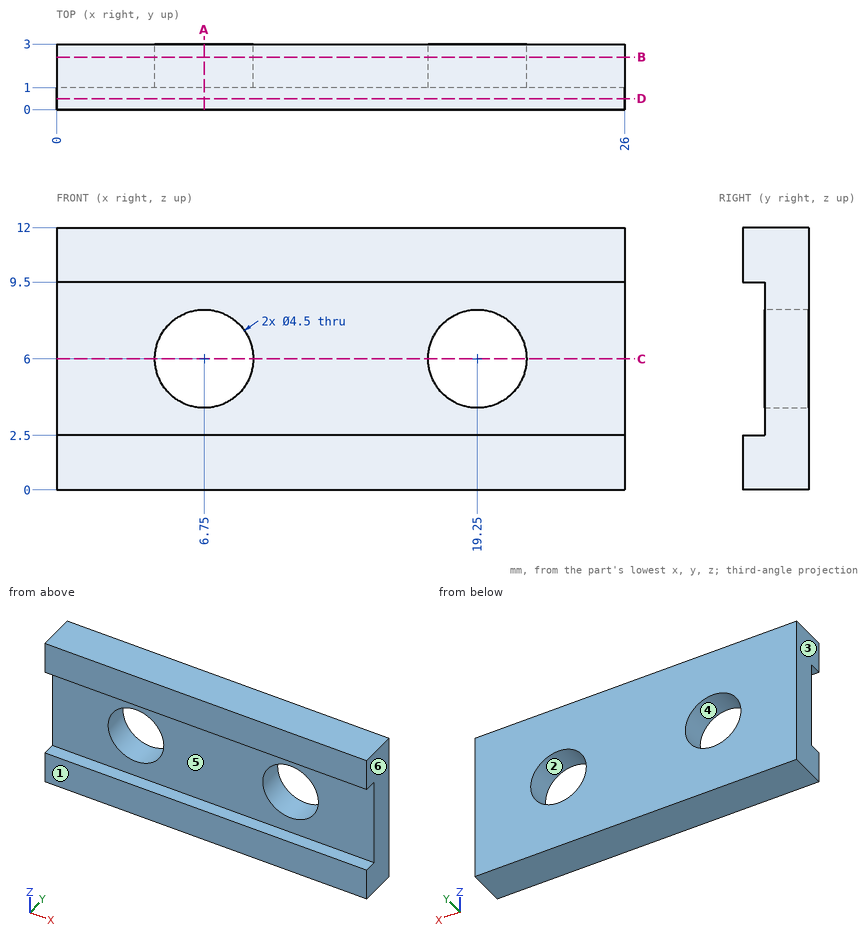
Job drawing, mm, ordinate dimensions from the low corner. One solid piece. A direction names the side the tool comes from. Coordinates: 2 decimals unless noted, no trailing zeros. Order: outer loops, then holes, each group sorted by start corner. A loop starts at its lowest first (then second) coordinate and runs counter-clockwise, first axis right, second up. Notation, with made-up numbers: (-22.75, 35.25) - (-13.75, 35.25) arc R31 ccw to (-13.75, 63.25) - close; hole circle Ø1 at (59, 83). An arc over 180 degrees is marked (long way). Use CSV: the item, a comma, the result in double quotes.
Item 1: Saw through at A-A on x = 6.75. Give the cut face in (y, z), and give its area (3 significant figures).
Solved:
outline,"(0, 0) - (3, 0) - (3, 3.75) - (1, 3.75) - (1, 2.5) - (0, 2.5) - close; (0, 9.5) - (1, 9.5) - (1, 8.25) - (3, 8.25) - (3, 12) - (0, 12) - close"
area,"20.0 mm²"
Item 2: Saw through at D-D on y = 0.5. Give the cut face in (x, z).
Solved:
outline,"(0, 0) - (26, 0) - (26, 2.5) - (0, 2.5) - close; (0, 9.5) - (26, 9.5) - (26, 12) - (0, 12) - close"
Item 3: Probe probe 1 along X at (y, z) = (2.5, 6); probe 2 along Z at (x, y) = (23.5, 0.25); probe 3 along X at (y, z) = (1.65, 6.75). List the from-to ranges inside material, lowest first.
Solved:
probe 1,"x = 0 to 4.5, 9 to 17, 21.5 to 26"
probe 2,"z = 0 to 2.5, 9.5 to 12"
probe 3,"x = 0 to 4.63, 8.87 to 17.13, 21.37 to 26"
Item 4: Mould opens along X. For the marked faces 1, 2, 3 and 4 say: +X half, -X half, draft (parallel to the pull), parting line (faces both ways), or undercut.
Solved:
face 1,"draft"
face 2,"undercut"
face 3,"-X half"
face 4,"undercut"
Item 5: Drop a flat-ended pin along its axis: P1, Ø5.5, axis at x = 11, z = 5.5, coming from the -Y side. Give the stop position or say it passes through.
Solved:
P1,"stops at y = 1"
Item 6: Saw through at C-C on z = 6. Give the cut face in (x, y).
Solved:
outline,"(0, 1) - (4.5, 1) - (4.5, 3) - (0, 3) - close; (9, 1) - (17, 1) - (17, 3) - (9, 3) - close; (21.5, 1) - (26, 1) - (26, 3) - (21.5, 3) - close"
Item 7: 3-axis set-ups, long thin cutter, end or side, ignore diameter. For the marked faces 5 and 6: which of +Z, -Z, +X, -X, +Y, -Y reach the whole face in a straight line?
Solved:
face 5,"+X, -X, -Y"
face 6,"+Z, -Z, +X, +Y, -Y"
Item 8: Saw through at B-B on y = 2.4. Give the cut face in (x, z).
Solved:
outline,"(0, 0) - (26, 0) - (26, 12) - (0, 12) - close; hole circle Ø4.5 at (6.75, 6); hole circle Ø4.5 at (19.25, 6)"
